Part model, mm, in its own coordinate system. A direction names the side the tool comes from. Coordinates: 2 decimals unless noted, no trailing zeros. Loops run counter-clockwise (first coordinate to the right, second up) from the corner with the lowest first, then second, coordinate; pieces in that order, holes last. Notation, with made-up numbers: (2, -5.5) -> (7, -5.5) arc R20 cw to (7, 25.5) -> close; hole circle Ø6 at (17.5, 13.5). An arc over 180 degrees is marked (long way). Use one line per item in the form item = value. Start each with the question number.
(1) Band-saw the part on A-A on z = 10. Give the cut face in (x, y), then the cut area to 3 significant figures.
(2) Band-saw the part on C-C on x = 43. Give the cut face in (y, z), then the cut area to 3 significant figures.
(3) Band-saw the part on B-B on y = 62. Give the cut face in (x, z).
(4) Band-saw the part on D-D on x = 65.5. Give the cut face in (y, z).
(5) Mould opens along X. For faces 1 (the cylindrical face through (41, 5, 10)), 2 (the flat face through (0, 49, 10)), 3 (the flat face through (42, 100, 3)) say: +X half, -X half, draft (parallel to the pull), parting line (faces both ways), or undercut.
(6) Drill centre lines: L1, parallel to X at y = 94.5, z = 6.25; L2, parallel to X at y = 7, z = 10; L3, parallel to Z at x = 77, y = 75. Where is each one in solid material? Low to high. Write a range as [from, to].
(7) 3-axis set-ups, long thin cutter, end or side, ignore diameter. For faces 4 (the flat face through (42, 51, 0)), 5 (the flat face through (42, 56, 5)): which of +Z, -Z, +X, -X, +Y, -Y reach the whole face in a straight line?
(8) Pin check, flat tips, straight feed: P1, Ø5, axis at x = 60, z = 9.5, coming from the +Y side; P2, Ø2.5, axis at x = 43, z = 10, coming from the -Y side. Stop position of each tip, or through.
```python
from build123d import *

# Parameters (mm, degrees)
SKETCH3_W           = 86
SKETCH3_H           = 100
BOSS_EXTRUDE1_DEPTH = 20
SKETCH5_W           = 76
SKETCH5_H           = 10
CUT_EXTRUDE1_DEPTH  = 90
SKETCH6_R           = 2
CUT_EXTRUDE2_DEPTH  = 90


with BuildPart() as part:
    # Sketch3 → Boss-Extrude1 (new body)
    with BuildSketch(Plane.XY):
        with Locations((43, 50)):
            Rectangle(SKETCH3_W, SKETCH3_H)
    extrude(amount=BOSS_EXTRUDE1_DEPTH)

    # Sketch5 → Cut-Extrude1 (cut)
    with BuildSketch(Plane(origin=(0, 100, 0), x_dir=(1, 0, 0), z_dir=(0, 1, 0))):
        with Locations((43, -10)):
            Rectangle(SKETCH5_W, SKETCH5_H)
    extrude(amount=-CUT_EXTRUDE1_DEPTH, mode=Mode.SUBTRACT)

    # Sketch6 → Cut-Extrude2 (cut)
    with BuildSketch(Plane(origin=(0, 10, 0), x_dir=(1, 0, 0), z_dir=(0, 1, 0))):
        with Locations(Location((43, -10, 0), (0, 0, 270))):
            Circle(SKETCH6_R)
    extrude(amount=-CUT_EXTRUDE2_DEPTH, mode=Mode.SUBTRACT)


solid = part.part
```
A:
q1.outline = (0, 0) -> (41, 0) -> (41, 10) -> (5, 10) -> (5, 100) -> (0, 100) -> close; (45, 0) -> (86, 0) -> (86, 100) -> (81, 100) -> (81, 10) -> (45, 10) -> close
q1.area = 1,720 mm²
q2.outline = (0, 0) -> (100, 0) -> (100, 5) -> (10, 5) -> (10, 8) -> (0, 8) -> close; (0, 12) -> (10, 12) -> (10, 15) -> (100, 15) -> (100, 20) -> (0, 20) -> close
q2.area = 1,060 mm²
q3.outline = (0, 0) -> (86, 0) -> (86, 20) -> (0, 20) -> close; hole (5, 5) -> (81, 5) -> (81, 15) -> (5, 15) -> close
q4.outline = (0, 0) -> (100, 0) -> (100, 5) -> (10, 5) -> (10, 15) -> (100, 15) -> (100, 20) -> (0, 20) -> close
q5.face_1 = undercut
q5.face_2 = -X half
q5.face_3 = draft
q6.L1 = [0, 5], [81, 86]
q6.L2 = [0, 41], [45, 86]
q6.L3 = [0, 5], [15, 20]
q7.face_4 = -Z, +X, -X, +Y, -Y
q7.face_5 = +Y
q8.P1 = 10
q8.P2 = through
